The model under review builds one solid part; all positions refer to its coordinate system, in mm. A direction names the side the tool comes from. Coordinates: 2 decimals unless noted, no trailing zeros. Loops run counter-clockwise (first coordinate to the right, second up) from the corner with the lowest first, then second, coordinate; pieces in that order, holes last. Notation, with made-up numbers: (80, 17) - (132, 17) arc R23 ccw to (132, 30) - close; hole circle Ø3 at (52, 57). An arc over 180 degrees is marked (long way). Use a Markdown table: item, result. Add a question column.
1) Add section D-D, the plane z = -7.5. Give the boundary of the cut face in (x, y), and give its area (3 significant figures).
2) Add section C-C, the plane y = 55. Give the boundary of the cut face in (x, z), and give its area (3 significant figures).
3) The part is to be moulded in two halves that separate along Z. For faces 1 (the flat face through (0, 0, 0)), 2 (the cylindrical face through (-10, 55.1, -17.5)), 3 (the flat face through (-9.965, 81.514, -26.415)), say which applies: pulls with the +Z half, pulls with the -Z half, needs draft (parallel to the pull), parting line crosses it, or undercut.
4) To check wall thickness, follow L1, parallel to Z at x = 8.65, y = 2.05; L2, parallel to Y at x = -8.95, z = 0; L3, parallel to X at y = 2, z = -7. State the ranges of each line that lie inside material, in increasing order. Write a range as [from, to].
5) Add section A-A, the plane x = -1.15. Give the boundary of the cut face in (y, z), and give its area (3 significant figures).
6) Clearance check with flat-ended pins moving along their axes: pin 1 (5 mm diameter, centred on x = 5.5, z = -1.5, fed in from +Y); pin 2 (12 mm diameter, centred on y = 75, z = -20, fed in from +X); pin 3 (5 mm diameter, centred on y = 9, z = -17.5, fed in from +X). State where each tip first meets the part, or that it passes through.
7) For faces 4 (the flat face through (4, 5, 0)), 5 (the flat face through (-12.5, 42, 0)), list the 3-axis set-ups (+Z, -Z, +X, -X, +Y, -Y) from which the entire face can be reached by the end or side of a thin tool; tool diameter is ignored.
8) Add section B-B, the plane z = 0. Give the boundary of the cut face in (x, y), and give its area (3 significant figures).
```python
from build123d import *

# Parameters (mm, degrees)
SKETCH1_W             = 25
SKETCH1_H             = 60
BOSS_EXTRUDE1_DEPTH   = 5
SKETCH8_W             = 5
SKETCH8_H             = 60
BOSS_EXTRUDE2_DEPTH   = 80
SKETCH9_R             = 2.5
CUT_EXTRUDE1_DEPTH    = 5
CUT_EXTRUDE2_REACH    = 7
FILLET1_R             = 2.5
F_3_0MM_DOWEL_HOLE2_D = 3
SKETCH15_R            = 2.5
CUT_EXTRUDE3_DEPTH    = 6


with BuildPart() as part:
    # Sketch1 → Boss-Extrude1 (new body)
    with BuildSketch(Plane(origin=(0, 0, 0), x_dir=(1, 0, 0), z_dir=(0, 1, 0))):
        Rectangle(SKETCH1_W, SKETCH1_H)
    extrude(amount=BOSS_EXTRUDE1_DEPTH)

    # Sketch8 → Boss-Extrude2 (add)
    with BuildSketch(Plane(origin=(0, 5, 0), x_dir=(1, 0, 0), z_dir=(0, 1, 0))):
        with Locations((-10, 0)):
            Rectangle(SKETCH8_W, SKETCH8_H)
    extrude(amount=BOSS_EXTRUDE2_DEPTH)

    # Sketch9 → Cut-Extrude1 (cut)
    with BuildSketch(Plane(origin=(-7.5, 0, 0), x_dir=(0, 0, -1), z_dir=(1, 0, 0))):
        with Locations((0, 55)):
            Circle(SKETCH9_R)
    extrude(amount=-CUT_EXTRUDE1_DEPTH, mode=Mode.SUBTRACT)

    # Sketch10 → Cut-Extrude2 (cut, up to next)
    with BuildSketch(Plane(origin=(-7.5, 0, 0), x_dir=(0, 0, -1), z_dir=(1, 0, 0)), mode=Mode.PRIVATE) as cut_extrude2_sk1:
        Polygon((-30, 77.928932188), (-22.928932188, 85), (-30, 85), align=None)
    cut_extrude2_tool1 = extrude(cut_extrude2_sk1.sketch, amount=-CUT_EXTRUDE2_REACH, mode=Mode.PRIVATE) & part.part
    add(cut_extrude2_tool1.solids().sort_by_distance((-7.5, 82.642977, 27.642977))[0], mode=Mode.SUBTRACT)
    # Sketch10 → Cut-Extrude2 (cut, up to next)
    with BuildSketch(Plane(origin=(-7.5, 0, 0), x_dir=(0, 0, -1), z_dir=(1, 0, 0)), mode=Mode.PRIVATE) as cut_extrude2_sk2:
        Polygon((22.928932188, 85), (30, 77.928932188), (30, 85), align=None)
    cut_extrude2_tool2 = extrude(cut_extrude2_sk2.sketch, amount=-CUT_EXTRUDE2_REACH, mode=Mode.PRIVATE) & part.part
    add(cut_extrude2_tool2.solids().sort_by_distance((-7.5, 82.642977, -27.642977))[0], mode=Mode.SUBTRACT)

    # Fillet1
    fillet1_edges = [part.edges().sort_by_distance(p)[0] for p in [
        (-7.5, 5, 0),
    ]]
    fillet(fillet1_edges, radius=FILLET1_R)

    # Ø3.0mm Dowel Hole2 (through all)
    with Locations(Plane(origin=(0, 5, 0), x_dir=(1, 0, 0), z_dir=(0, 1, 0))):
        with Locations((-1.15, -7.5), (-1.15, 7.5)):
            f_3_0mm_dowel_hole2 = Hole(F_3_0MM_DOWEL_HOLE2_D / 2)

    # Mirror1: Ø3.0mm Dowel Hole2 across plane
    add(f_3_0mm_dowel_hole2.mirror(Plane(origin=(3.75, 0, 0), x_dir=(0, 0, 1), z_dir=(1, 0, 0))), mode=Mode.SUBTRACT)

    # Sketch15 → Cut-Extrude3 (cut, through all)
    with BuildSketch(Plane(origin=(-7.5, 0, 0), x_dir=(0, 0, -1), z_dir=(1, 0, 0))):
        with Locations((20, 55)):
            Circle(SKETCH15_R)
    extrude(amount=-CUT_EXTRUDE3_DEPTH, mode=Mode.SUBTRACT)


solid = part.part
```
From the geometry:
| question | item | result |
|---|---|---|
| 1 | outline | (-12.5, 0) - (-2.65, 0) - (-2.65, 5) - (-5, 5) arc R2.5 cw to (-7.5, 7.5) - (-7.5, 85) - (-12.5, 85) - close; (0.35, 0) - (7.15, 0) - (7.15, 5) - (0.35, 5) - close; (10.15, 0) - (12.5, 0) - (12.5, 5) - (10.15, 5) - close |
| 1 | area | 496 mm^2 |
| 2 | outline | (-12.5, -30) - (-7.5, -30) - (-7.5, -22.5) - (-12.5, -22.5) - close; (-12.5, -17.5) - (-7.5, -17.5) - (-7.5, -2.5) - (-12.5, -2.5) - close; (-12.5, 2.5) - (-7.5, 2.5) - (-7.5, 30) - (-12.5, 30) - close |
| 2 | area | 250 mm^2 |
| 3 | face 1 | needs draft |
| 3 | face 2 | undercut |
| 3 | face 3 | pulls with the -Z half |
| 4 | L1 | z = [-30, -9], [-6, 6], [9, 30] |
| 4 | L2 | y = [0, 52.5], [57.5, 85] |
| 4 | L3 | x = [-12.5, -2.56], [0.26, 7.24], [10.06, 12.5] |
| 5 | outline | (0, -30) - (5, -30) - (5, -9) - (0, -9) - close; (0, -6) - (5, -6) - (5, 6) - (0, 6) - close; (0, 9) - (5, 9) - (5, 30) - (0, 30) - close |
| 5 | area | 270 mm^2 |
| 6 | pin 1 | stops at y = 5 |
| 6 | pin 2 | stops at x = -7.5 |
| 6 | pin 3 | stops at x = -7.29 |
| 7 | face 4 | +Z, -Z, +X, +Y |
| 7 | face 5 | +Z, -Z, -X, +Y, -Y |
| 8 | outline | (-12.5, 0) - (12.5, 0) - (12.5, 5) - (-5, 5) arc R2.5 cw to (-7.5, 7.5) - (-7.5, 52.5) - (-12.5, 52.5) - close; (-12.5, 57.5) - (-7.5, 57.5) - (-7.5, 85) - (-12.5, 85) - close |
| 8 | area | 501 mm^2 |
